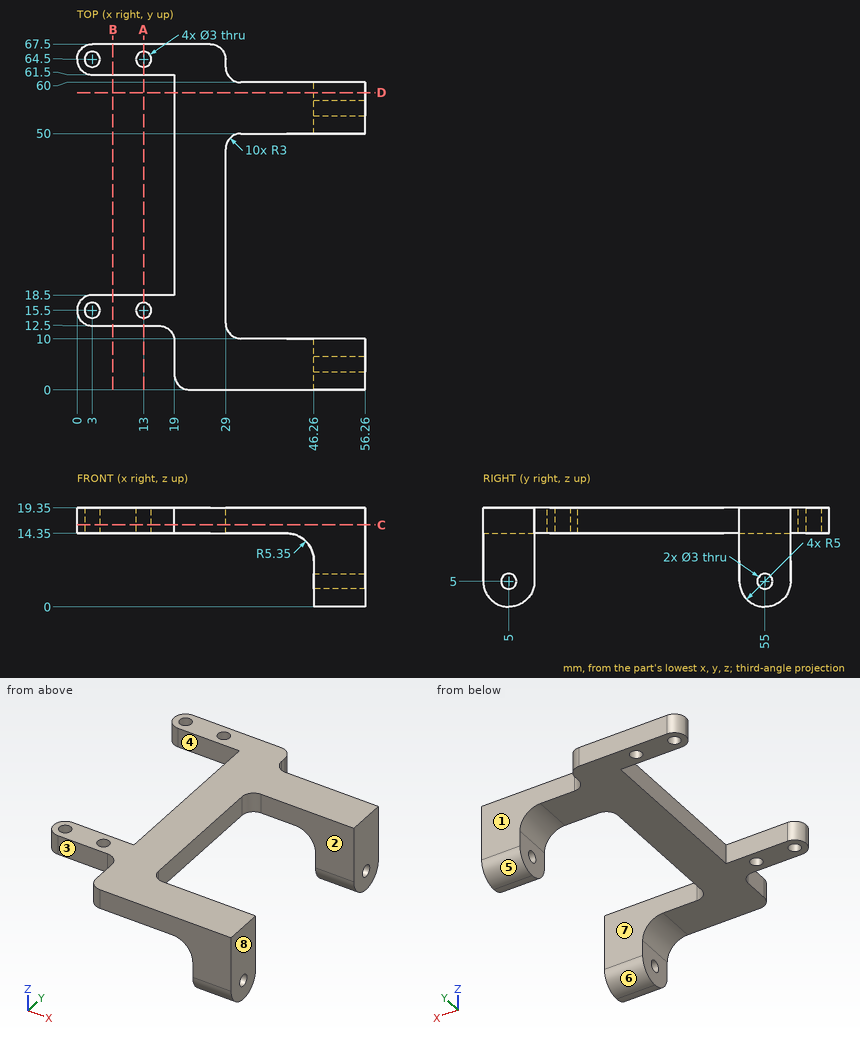
Could you check a few things on this drawing? It's one solid part, dimensions in mm from its lowest x, y, z. A direction names the side the tool comes from. Give positions to 0.01 mm unless a question says otherwise; leave off trailing zeros. Order: outer loops, then holes, each group sorted by start corner. A loop starts at its lowest first (then second) coordinate and runs counter-clockwise, first axis right, second up. Notation, with made-up numbers: (23.25, -30.5) - (59.25, -30.5) arc R13 ccw to (59.25, -24.5) - close; hole circle Ø7 at (-7, 9). An arc over 180 degrees is marked (long way). One line per item, written item: value. Start each with the question number.
1. If I drill on probe 1 along X at (y, z) = (64.5, 17.8); probe 2 along Y at (x, z) = (3, 17.5); probe 3 along Y at (x, z) = (49.25, 5), over which ranges is the centre line in solid material (lowest first)?
2. Imagine slicing it at C-C on z = 16. Give the number of separate pieces and of enclosed holes in the cut face, plus the area to 3 significant figures.
3. Imagine slicing it at B-B on x = 7. List the corners of the cut face in (y, z) for me.
4. For P1, Ø0.5, axis at y = 64, z = 16.5, coming from the +X side; P2, Ø2.5, axis at y = 41.5, z = 15.5, coming from the -X side; P3, Ø4.5, axis at y = 54.5, z = 2.5, coming from the -X side; P4, Ø2.5, axis at x = 3, y = 15.5, coming from the +Z side, each with a flat end and sliding along its axis, tell me the tip position at first contact or that it passes through.
5. Imagine slicing it at A-A on x = 13. List the corners of the cut face in (y, z) for me, plus the area to 3 significant figures.
6. For the marked faces 1, 2, 3 and 4, which set-ups out of +Z, -Z, +X, -X, +Y, -Y let a thin tool reach every point of the face, with its end or its side?
7. Thinking about a two-plate mould opening in Y: for the marked faces 5, 6, 7 and 8, which applies, +Y half, -Y half, draft (parallel to the pull), parting line (faces both ways), or undercut?
8. Imagine slicing it at D-D on y = 58. List the corners of the cut face in (x, z) for me.
Values:
1. probe 1: 0 to 1.5, 4.5 to 11.5, 14.5 to 29
1. probe 2: 12.5 to 14, 17 to 18.5, 61.5 to 63, 66 to 67.5
1. probe 3: 0 to 3.5, 6.5 to 10, 50 to 53.5, 56.5 to 60
2. separate pieces: 1
2. enclosed holes: 4
2. area: 1,420 mm²
3. outline: (12.5, 14.35) - (18.5, 14.35) - (18.5, 19.35) - (12.5, 19.35) - close; (61.5, 14.35) - (67.5, 14.35) - (67.5, 19.35) - (61.5, 19.35) - close
4. P1: x = 29
4. P2: x = 19
4. P3: x = 46.26
4. P4: through
5. outline: (12.5, 14.35) - (14, 14.35) - (14, 19.35) - (12.5, 19.35) - close; (17, 14.35) - (18.5, 14.35) - (18.5, 19.35) - (17, 19.35) - close; (61.5, 14.35) - (63, 14.35) - (63, 19.35) - (61.5, 19.35) - close; (66, 14.35) - (67.5, 14.35) - (67.5, 19.35) - (66, 19.35) - close
5. area: 30.0 mm²
6. face 1: +Z, -Z, +X, +Y
6. face 2: +Z, -Z, +X
6. face 3: +Z, -Z, -X, -Y
6. face 4: +Z, -Z, -X
7. face 5: +Y half
7. face 6: undercut
7. face 7: undercut
7. face 8: draft
8. outline: (19, 14.35) - (40.91, 14.35) arc R5.35 cw to (46.26, 9) - (46.26, 1) - (56.26, 1) - (56.26, 19.35) - (19, 19.35) - close
